Geometry check sheet. Reference: drawing and pictorial views, mm from the part's lowest x, y, z. Round coordinates to 2 decimals unless told otherwise and drop trailing zeros.
Q1. Depth check by flat-ended pin: P1, Ø2.5, axis at x = 49.5, y = 14.5, coming from the +Z side; P2, Ø1.2, axis at x = 3, y = 14.5, coming from the -Z side. Enter the tip coordinate at first touch or a pass-through.
Q2. Cross-section at A-A on z = 1.55. Give the number of separate pieces and of enclosed holes in the cut face, then the cut area to 3 significant figures.
Q3. Scan lines: probe 1 along Y at (x, z) = (7.5, 1.1); probe 2 along Y at (x, z) = (78, 1.2); probe 3 along Y at (x, z) = (45.5, 0.9). Record each from-to range of solid material in increasing order.
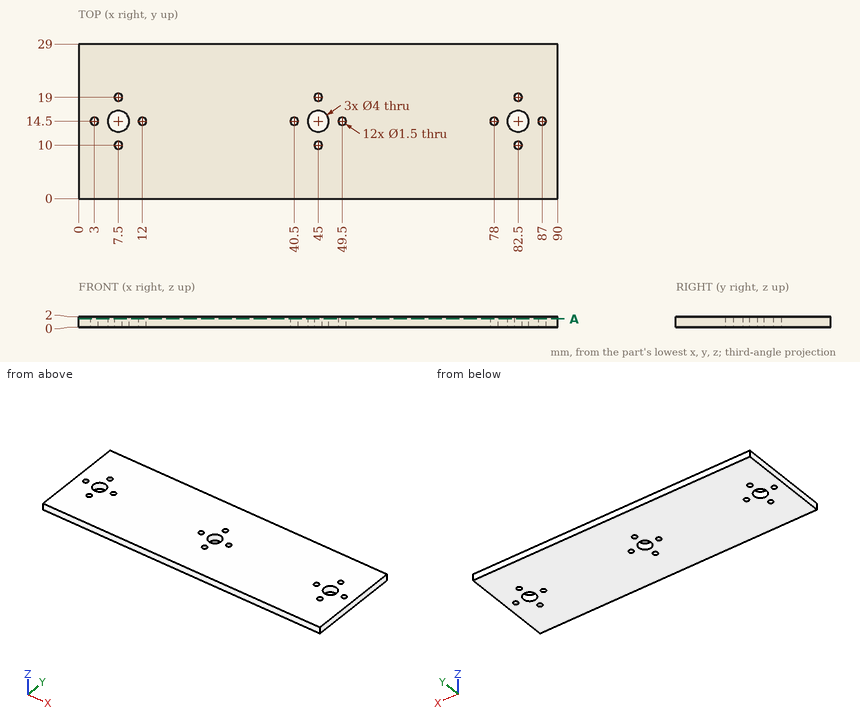
Results found:
1. P1: stops at z = 2
1. P2: passes through
2. separate pieces: 1
2. enclosed holes: 15
2. area: 2,550 mm2
3. probe 1: y = 0 to 9.25, 10.75 to 12.5, 16.5 to 18.25, 19.75 to 29
3. probe 2: y = 0 to 13.75, 15.25 to 29
3. probe 3: y = 0 to 9.44, 10.56 to 12.56, 16.44 to 18.44, 19.56 to 29
